Check sheet for the modelled part. Datum: model origin and axes. Units: mm. Face numbers are marked on the shaded views. Give positions to 0.01 mm unless a question says otherwise; leave off trailing zeros. Order: outer loops, then holes, each group sorted by start corner. A loop starts at its lowest first (then second) coordinate and runs counter-clockwise, first axis right, second up.
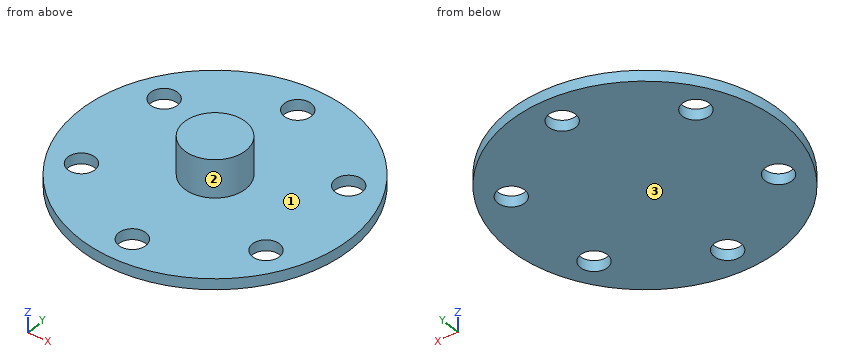
```python
from build123d import *

# Parameters (mm, degrees)
SKETCH4_R           = 63.5
BOSS_EXTRUDE1_DEPTH = 5.08
SKETCH5_R           = 14.351
BOSS_EXTRUDE2_DEPTH = 17.78
SKETCH6_R           = 6.35
CUT_EXTRUDE1_DEPTH  = 17.78


with BuildPart() as part:
    # Sketch4 → Boss-Extrude1 (new body)
    with BuildSketch(Plane.XY):
        Circle(SKETCH4_R)
    extrude(amount=-BOSS_EXTRUDE1_DEPTH)

    # Sketch5 → Boss-Extrude2 (add)
    with BuildSketch(Plane.XY):
        Circle(SKETCH5_R)
    extrude(amount=BOSS_EXTRUDE2_DEPTH)

    # Sketch6 → Cut-Extrude1 (cut)
    with BuildSketch(Plane.XY):
        with Locations((0, 49.784)):
            Circle(SKETCH6_R)
        with Locations((43.114208702, 24.892)):
            Circle(SKETCH6_R)
        with Locations((43.114208702, -24.892)):
            Circle(SKETCH6_R)
        with Locations((0, -49.784)):
            Circle(SKETCH6_R)
        with Locations((-43.114208702, -24.892)):
            Circle(SKETCH6_R)
        with Locations((-43.114208702, 24.892)):
            Circle(SKETCH6_R)
    extrude(amount=-CUT_EXTRUDE1_DEPTH, mode=Mode.SUBTRACT)


solid = part.part
```
(1) Cross-section at C-C on y = -45. Enter the section's corners in (x, z), then the cut area to 3 significant figures.
Response values:
outline: (-44.8, -5.08) - (-4.18, -5.08) - (-4.18, 0) - (-44.8, 0) - close; (4.18, -5.08) - (44.8, -5.08) - (44.8, 0) - (4.18, 0) - close
area: 413 mm2
(2) Cross-section at D-D on z = 15.25. Enter the section's corners in (x, y), then the cut area to 3 significant figures.
Response values:
outline: circle Ø28.7 at (0, 0)
area: 647 mm2
(3) Cross-section at B-B on y = 0. Enter the section's corners in (x, z).
Response values:
outline: (-63.5, -5.08) - (63.5, -5.08) - (63.5, 0) - (14.35, 0) - (14.35, 17.78) - (-14.35, 17.78) - (-14.35, 0) - (-63.5, 0) - close
(4) Gauge pin test, flat ends, axial feed: pin 1 Ø6 at (x, y) = (18.5, 31.5) entering from +Z; pin 2 Ø5 at (x, z) = (7.5, 6) entering from -Y; pin 3 Ø10 at (x, y) = (0, -49.784) entering from -Z; pin 4 Ø12 at (x, z) = (-30.5, 1.5) entering from -Y. Record the tip position at first contact, or that the pin passes through.
Response values:
pin 1: stops at z = 0
pin 2: stops at y = -13.45
pin 3: passes through
pin 4: stops at y = -58.5
(5) Material ranges on L1, parallel to Y at x = 0, z = -2.7; L2, parallel to X at y = -26.5, z = -2; L3, parallel to Z at x = 17, y = 48, recorded low to high.
Response values:
L1: y = -63.5 to -56.13, -43.43 to 43.43, 56.13 to 63.5
L2: x = -57.71 to -49.26, -36.97 to 36.97, 49.26 to 57.71
L3: z = -5.08 to 0
(6) Cross-section at A-A on x = 0. Enter the section's corners in (y, z), then the cut area to 3 significant figures.
Response values:
outline: (-63.5, -5.08) - (-56.13, -5.08) - (-56.13, 0) - (-63.5, 0) - close; (-43.43, -5.08) - (43.43, -5.08) - (43.43, 0) - (14.35, 0) - (14.35, 17.78) - (-14.35, 17.78) - (-14.35, 0) - (-43.43, 0) - close; (56.13, -5.08) - (63.5, -5.08) - (63.5, 0) - (56.13, 0) - close
area: 1,030 mm2
(7) Release check for a two-part mould opening along Z. For the marked faces 1, 2 and 3 record: released by +Z, released by -Z, zero draft, split by the parting line, or undercut.
Response values:
face 1: released by +Z
face 2: zero draft
face 3: released by -Z
